Can you work these out from the drawing? Everything is in mm from the part's minimum corner. Give positions to 0.01 mm unless a question says otherwise; leave off trailing zeros. Loops run counter-clockwise (first coordinate to the right, second up) from the corner with the lowest first, then second, coordinate; pieces in that order, holes last. Notation, with made-up numbers: (88.5, 53.25) -> (146.5, 53.25) arc R18 ccw to (146.5, 79.25) -> close; hole circle Ø3 at (-20.5, -13). An arc over 180 degrees is marked (long way). Write item = value, one per line. Start each with the question number.
1) I'm going to push flat-ended pins straight in: pin 1 Ø1.5 at (x, z) = (20, 30) entering from -Y; pin 2 Ø10 at (x, z) = (66.5, 8.5) entering from -Y; pin 3 Ø2 at (x, y) = (48, 11) entering from +Z; pin 4 Ø1 at (x, z) = (11.5, 23) entering from -Y. Where does each tip first touch, or does it pass through?
2) I want a section at C-C (y = 62.5). List the corners of the cut face in (x, z) for me (3 decimals).
3) I need wall thicknesses on probe 1 along Z at (x, y) = (38, 49); probe 2 along Z at (x, y) = (28.5, 28); probe 3 along X at (y, z) = (12, 30). Which ranges of each line are inside material? Lowest first, please. Write a range as from..to.
4) If we mould it in two halves opening along X, with no side actions, what happens to the marked faces 1, 2 and 3? For each: +X half, -X half, draft (parallel to the pull), parting line (faces both ways), or undercut.
5) I want a section at B-B (z = 38.1). List the corners of the cut face in (x, y) for me (3 decimals).
6) I want a section at A-A (x = 38.1). List the corners of the cut face in (y, z) for me (3 decimals), and give its area (3 significant figures).
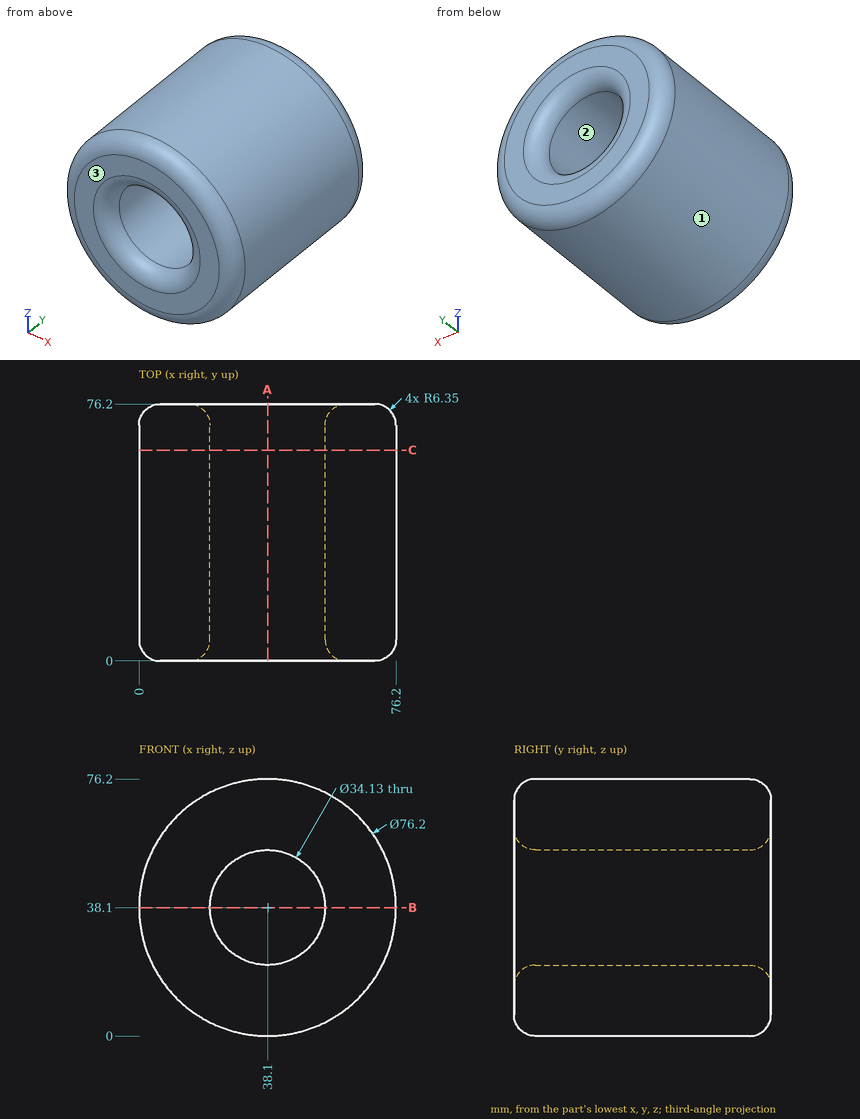
Answer list:
q1.pin_1 = 0.67
q1.pin_2 = 1.65
q1.pin_3 = 75.15
q1.pin_4 = 0
q2.outline = circle Ø76.2 at (38.1, 38.1); hole circle Ø34.13 at (38.1, 38.1)
q3.probe_1 = 0..21.04, 55.16..76.2
q3.probe_2 = 1.23..23.99, 52.21..74.97
q3.probe_3 = 0.87..23.08, 53.12..75.33
q4.face_1 = parting line
q4.face_2 = undercut
q4.face_3 = draft
q5.outline = (0, 6.35) arc R6.35 ccw to (6.35, 0) -> (14.685, 0) arc R6.35 ccw to (21.035, 6.35) -> (21.035, 69.85) arc R6.35 ccw to (14.685, 76.2) -> (6.35, 76.2) arc R6.35 ccw to (0, 69.85) -> close; (55.165, 6.35) arc R6.35 ccw to (61.515, 0) -> (69.85, 0) arc R6.35 ccw to (76.2, 6.35) -> (76.2, 69.85) arc R6.35 ccw to (69.85, 76.2) -> (61.515, 76.2) arc R6.35 ccw to (55.165, 69.85) -> close
q6.outline = (0, 6.35) arc R6.35 ccw to (6.35, 0) -> (69.85, 0) arc R6.35 ccw to (76.2, 6.35) -> (76.2, 14.685) arc R6.35 ccw to (69.85, 21.035) -> (6.35, 21.035) arc R6.35 ccw to (0, 14.685) -> close; (0, 61.515) arc R6.35 ccw to (6.35, 55.165) -> (69.85, 55.165) arc R6.35 ccw to (76.2, 61.515) -> (76.2, 69.85) arc R6.35 ccw to (69.85, 76.2) -> (6.35, 76.2) arc R6.35 ccw to (0, 69.85) -> close
q6.area = 3,140 mm^2
